Source: CAD feature listing. Evaluate the final solid. Frame: model axes, mm. Give positions to 0.01 mm unless a question says otherwise; leave off trailing zeros. Order: outer loops, then holes, each group sorted by start corner. A loop starts at its lowest first (then second) coordinate and runs counter-clockwise, first axis right, second up.
from build123d import *

# Parameters (mm, degrees)
F1_DEPTH = 1.5875


with BuildPart() as f1:
    # F0 (on Front) → F1 (new body)
    with BuildSketch(Plane.XZ):
        with BuildLine():
            ThreePointArc((15.7750619272, 15.6556075), (17.2957745251, 18.7170405077), (18.2286550123, 22.0056075))
            ThreePointArc((18.2286550123, 22.0056075), (9.6881471574, 26.8825301945), (0, 28.575))
            Line((0, 28.575), (0, 26.9875))
            ThreePointArc((0, 26.9875), (1.1225320151, 26.5225320151), (1.5875, 25.4))
            ThreePointArc((1.5875, 25.4), (1.1225320151, 24.2774679849), (0, 23.8125))
            Line((0, 23.8125), (0, 22.225))
            ThreePointArc((0, 22.225), (8.5441426812, 20.5170234402), (15.7750619272, 15.6556075))
        make_face()
        with BuildLine():
            Line((0, 26.9875), (0, 28.575))
            ThreePointArc((0, 28.575), (-17.0243221699, -22.9500126287), (27.3461703442, 8.2896075))
            ThreePointArc((27.3461703442, 8.2896075), (24.9460595827, 4.9482842946), (22.140202071, 1.9396075))
            ThreePointArc((22.140202071, 1.9396075), (-15.0140409003, -16.3868606159), (0, 22.225))
            Line((0, 22.225), (0, 23.8125))
            ThreePointArc((0, 23.8125), (-1.5875, 25.4), (0, 26.9875))
        make_face()
        with BuildLine():
            ThreePointArc((0, 6.858), (9.0312025297, 9.2060769155), (15.7750619272, 15.6556075))
            ThreePointArc((15.7750619272, 15.6556075), (8.5441426812, 20.5170234402), (0, 22.225))
            Line((0, 22.225), (0, 6.858))
        make_face()
        with BuildLine():
            Line((0, 6.858), (0, 22.225))
            ThreePointArc((0, 22.225), (-15.0140409003, -16.3868606159), (22.140202071, 1.9396075))
            ThreePointArc((22.140202071, 1.9396075), (11.9120364072, -4.5780244952), (0, -6.858))
            ThreePointArc((0, -6.858), (-6.858, 0), (0, 6.858))
        make_face()
    extrude(amount=F1_DEPTH)


solid = f1.part
1) Ray query, L1, parallel to Z at x = 8, y = -0.25; L2, parallel to X at y = -0.3, z = -4; L3, parallel to Z at x = 12, y = -0.9. Return the intervals inside material, ascending.
Checks:
L1: z = -27.43 to -5.85, 8.67 to 27.43
L2: x = -28.29 to -5.57, 13.27 to 28.29
L3: z = -25.93 to -4.54, 11.26 to 25.93
2) Section query C-C on z = 12. Output: boundary loops of the cut face in (x, y).
Checks:
outline: (-25.93, -1.59) - (12.82, -1.59) - (12.82, 0) - (-25.93, 0) - close
3) Pull-direction query (X, two-part tool) for faces 1 (the face through (-6.856, -0.783, -0.151)), 2 (the face through (-7, 0, -6)); classes: +X half, -X half, draft (parallel to the pull), parting line (faces both ways), or undercut.
Checks:
face 1: undercut
face 2: draft
4) Section query B-B on z = 0. Output: boundary loops of the cut face in (x, y) (1 decimal), and give its area (3 significant figures).
Checks:
outline: (-28.6, -1.6) - (-6.9, -1.6) - (-6.9, 0) - (-28.6, 0) - close; (19.9, -1.6) - (28.6, -1.6) - (28.6, 0) - (19.9, 0) - close
area: 48.3 mm2
5) Section query D-D on z = -15. Output: boundary loops of the cut face in (x, y).
Checks:
outline: (-24.32, -1.59) - (24.32, -1.59) - (24.32, 0) - (-24.32, 0) - close
